Build history of the part. All positions in model axes, mm. A direction names the side the tool comes from. Round coordinates to 2 decimals unless told otherwise and drop trailing zeros. Write each loop counter-clockwise with the first axis right and the second up, starting at its lowest first coordinate (ties: lowest second). Pieces come first, ordered by that corner, then holes.
from build123d import *

# Parameters (mm, degrees)
SKETCH1_W               = 17.5
SKETCH1_H               = 80
BOSS_EXTRUDE1_DEPTH     = 100
BOSS_EXTRUDE1_2_DEPTH   = 100
SKETCH2_W               = 70
SKETCH2_H               = 80
BOSS_EXTRUDE2_DEPTH     = 20
CUT_EXTRUDE1_DEPTH      = 145.568322948
CUT_EXTRUDE1_DEPTH_BACK = 145.568322948
SKETCH5_R               = 11.25
CUT_EXTRUDE2_DEPTH      = 145.568322948
CUT_EXTRUDE2_DEPTH_BACK = 145.568322948
SKETCH6_W               = 42.5
SKETCH6_H               = 42.5
CUT_EXTRUDE3_DEPTH      = 7.5
SKETCH7_R               = 1.75
CUT_EXTRUDE4_DEPTH      = 145.568322948
CUT_EXTRUDE4_DEPTH_BACK = 145.568322948
SKETCH8_W               = 42.5
SKETCH8_H               = 42.5
CUT_EXTRUDE5_DEPTH      = 7.5
CUT_EXTRUDE7_DEPTH      = 35
SKETCH10_W              = 47.5
SKETCH10_H              = 15
BOSS_EXTRUDE3_DEPTH     = 47.5
SKETCH11_R              = 11.25
SKETCH11_R_2            = 1.75
CUT_EXTRUDE8_DEPTH      = 142.089510595
SKETCH12_W              = 42.5
SKETCH12_H              = 42.5
CUT_EXTRUDE9_DEPTH      = 5
SKETCH13_R              = 17.5
BOSS_EXTRUDE4_DEPTH     = 20
FILLET1_R               = 10


with BuildPart() as part:
    # Sketch1 → Boss-Extrude1 (new body)
    with BuildSketch(Plane.XY):
        with Locations((-26.25, 0)):
            Rectangle(SKETCH1_W, SKETCH1_H)
    extrude(amount=BOSS_EXTRUDE1_DEPTH)



with BuildPart() as body_2:
    # Sketch1 → Boss-Extrude1 2 (new body)
    with BuildSketch(Plane.XY):
        with Locations((26.25, 0)):
            Rectangle(SKETCH1_W, SKETCH1_H)
    extrude(amount=BOSS_EXTRUDE1_2_DEPTH)


with BuildPart() as part_1:
    add(part.part)

    add(body_2.part)  # Boss-Extrude2 merges body 2
    # Sketch2 → Boss-Extrude2 (add)
    with BuildSketch(Plane.XY.offset(100)):
        Rectangle(SKETCH2_W, SKETCH2_H)
    extrude(amount=BOSS_EXTRUDE2_DEPTH)

    # Sketch3 → Cut-Extrude1 (cut, two sides)
    with BuildSketch(Plane(origin=(35, 0, 0), x_dir=(0, 0, -1), z_dir=(1, 0, 0))) as cut_extrude1_sk:
        with BuildLine():
            ThreePointArc((-55, 0), (-40, -15), (-25, 0))
            Line((-25, 0), (-55, 0))
        make_face()
        with BuildLine():
            Line((-55, 0), (-25, 0))
            ThreePointArc((-25, 0), (-40, 15), (-55, 0))
        make_face()
        with BuildLine():
            ThreePointArc((-40, 40), (-11.715728753, 28.284271247), (0, 0))
            Line((0, 0), (0, 40))
            Line((0, 40), (-40, 40))
        make_face()
        with BuildLine():
            Line((0, -40), (0, 0))
            ThreePointArc((0, 0), (-11.715728753, -28.284271247), (-40, -40))
            Line((-40, -40), (0, -40))
        make_face()
    extrude(amount=CUT_EXTRUDE1_DEPTH, mode=Mode.SUBTRACT)
    extrude(cut_extrude1_sk.sketch, amount=-CUT_EXTRUDE1_DEPTH_BACK, mode=Mode.SUBTRACT)

    # Sketch5 → Cut-Extrude2 (cut, two sides)
    with BuildSketch(Plane.ZY.offset(35)) as cut_extrude2_sk:
        with Locations(Location((90, 0, 0), (0, 0, 270))):
            Circle(SKETCH5_R)
    extrude(amount=CUT_EXTRUDE2_DEPTH, mode=Mode.SUBTRACT)
    extrude(cut_extrude2_sk.sketch, amount=-CUT_EXTRUDE2_DEPTH_BACK, mode=Mode.SUBTRACT)

    # Sketch6 → Cut-Extrude3 (cut)
    with BuildSketch(Plane(origin=(35, 0, 0), x_dir=(0, 0, -1), z_dir=(1, 0, 0))):
        with Locations((-90, 0)):
            Rectangle(SKETCH6_W, SKETCH6_H)
    extrude(amount=-CUT_EXTRUDE3_DEPTH, mode=Mode.SUBTRACT)

    # Sketch7 → Cut-Extrude4 (cut, two sides)
    with BuildSketch(Plane(origin=(35, 0, 0), x_dir=(0, 0, -1), z_dir=(1, 0, 0))) as cut_extrude4_sk:
        with Locations((-105.5, 15.5)):
            Circle(SKETCH7_R)
        with Locations((-74.5, 15.5)):
            Circle(SKETCH7_R)
        with Locations((-74.5, -15.5)):
            Circle(SKETCH7_R)
        with Locations((-105.5, -15.5)):
            Circle(SKETCH7_R)
    extrude(amount=CUT_EXTRUDE4_DEPTH, mode=Mode.SUBTRACT)
    extrude(cut_extrude4_sk.sketch, amount=-CUT_EXTRUDE4_DEPTH_BACK, mode=Mode.SUBTRACT)

    # Sketch8 → Cut-Extrude5 (cut)
    with BuildSketch(Plane.ZY.offset(35)):
        with Locations((90, 0)):
            Rectangle(SKETCH8_W, SKETCH8_H)
    extrude(amount=-CUT_EXTRUDE5_DEPTH, mode=Mode.SUBTRACT)

    # Sketch9 → Cut-Extrude7 (cut)
    with BuildSketch(Plane.ZY.offset(-17.5)):
        with BuildLine():
            Line((105.5, 19.25), (95.963116285, 19.25))
            Line((95.963116285, 19.25), (95.963116285, 11.75))
            Line((95.963116285, 11.75), (105.5, 11.75))
            ThreePointArc((105.5, 11.75), (109.25, 15.5), (105.5, 19.25))
        make_face()
        with BuildLine():
            Line((105.5, -11.75), (95.963116285, -11.75))
            Line((95.963116285, -11.75), (95.963116285, -19.25))
            Line((95.963116285, -19.25), (105.5, -19.25))
            ThreePointArc((105.5, -19.25), (109.25, -15.5), (105.5, -11.75))
        make_face()
    extrude(amount=CUT_EXTRUDE7_DEPTH, mode=Mode.SUBTRACT)

    # Sketch10 → Boss-Extrude3 (add)
    with BuildSketch(Plane(origin=(0, 40, 0), x_dir=(1, 0, 0), z_dir=(0, 1, 0))):
        with Locations((0, -112.5)):
            Rectangle(SKETCH10_W, SKETCH10_H)
    extrude(amount=BOSS_EXTRUDE3_DEPTH)

    # Sketch11 → Cut-Extrude8 (cut, through all)
    with BuildSketch(Plane(origin=(0, 0, 105), x_dir=(-1, 0, 0), z_dir=(0, 0, -1))):
        with Locations((0, 63.75)):
            Circle(SKETCH11_R)
        with Locations((15.5, 79.25)):
            Circle(SKETCH11_R_2)
        with Locations((15.5, 48.25)):
            Circle(SKETCH11_R_2)
        with Locations((-15.5, 48.25)):
            Circle(SKETCH11_R_2)
        with Locations((-15.5, 79.25)):
            Circle(SKETCH11_R_2)
    extrude(amount=-CUT_EXTRUDE8_DEPTH, mode=Mode.SUBTRACT)

    # Sketch12 → Cut-Extrude9 (cut)
    with BuildSketch(Plane(origin=(0, 0, 105), x_dir=(-1, 0, 0), z_dir=(0, 0, -1))):
        with Locations((0, 63.75)):
            Rectangle(SKETCH12_W, SKETCH12_H)
    extrude(amount=-CUT_EXTRUDE9_DEPTH, mode=Mode.SUBTRACT)

    # Sketch13 → Boss-Extrude4 (add)
    with BuildSketch(Plane.XY.offset(120)):
        with Locations(Location((0, 0, 0), (0, 0, 180))):
            Circle(SKETCH13_R)
    extrude(amount=BOSS_EXTRUDE4_DEPTH)

    # Fillet1
    fillet1_edges = [part_1.edges().sort_by_distance(p)[0] for p in [
        (-17.5, -40, 70),
        (-17.5, 40, 70),
        (17.5, 0, 0),
        (-17.5, 0, 0),
        (17.5, -40, 70),
        (17.5, 40, 70),
    ]]
    fillet(fillet1_edges, radius=FILLET1_R)


solid = part_1.part
1) Which spindle directions (+Z, -Z, +X, -X, +Y, -Y) get a long thin tool onto all of the face, cutting with end or side? Do faces 4 (the cylindrical face through (-20.51, 37.15, 69.58)), 5 (the cylindrical face through (0.25, 15.42, 109.25)), 6 (the flat face through (31, 0, 111.25)), 7 (the flat face through (-2, 87, 105)). Say none if no direction does.
Results:
face 4: -Z, +Y
face 5: -Z
face 6: +X
face 7: -Z, +X, -X, +Y
2) Mould opens along Z. For faces 1 (the flat face through (0, 85, 107)), 2 (the cylindrical face through (0.25, -15.58, 109.25)), 3 (the flat face through (-27.5, -9, 99)) say: released by +Z, released by -Z, zero draft, split by the parting line, or undercut.
Results:
face 1: zero draft
face 2: released by -Z
face 3: undercut
3) Slice it at D-D (x = -15.5). Count the separate pieces of the cut face and the enclosed holes in it, plus the area to 3 significant figures.
Results:
separate pieces: 3
enclosed holes: 0
area: 2,220 mm2
4) Slice it at B-B (x = -30). Write the cut outline in (y, z).
Results:
outline: (-40, 40) arc R40 ccw to (40, 40) - (40, 120) - (-40, 120) - close; hole (-21.25, 68.75) - (21.25, 68.75) - (21.25, 111.25) - (-21.25, 111.25) - close; hole circle Ø30 at (0, 40)
5) Pin check, flat tips, straight feed: pin 1 Ø10 at (x, y) = (13.5, 67.5) entering from +Z; pin 2 Ø3 at (x, y) = (-2.5, 6) entering from -Z; pin 3 Ø3 at (y, z) = (-15.5, 105.5) entering from +X; pin 4 Ø2 at (x, z) = (-17.5, 93.5) entering from +Y. Stop position of each tip, or through.
Results:
pin 1: stops at z = 120
pin 2: stops at z = 100
pin 3: passes through
pin 4: stops at y = 34.36
6) Wall check: L1, parallel to Y at x = -24, z = 105.5; L2, parallel to Y at x = -15.5, z = 115.5; L3, parallel to Z at x = -20, y = 0.5. Give the ranges that are in metal, low to high.
Results:
L1: y = -40 to -17.25, -13.75 to 13.75, 17.25 to 40
L2: y = -40 to 46.5, 50 to 77.5, 81 to 87.5
L3: z = 3.39 to 25.01, 54.99 to 78.76, 101.24 to 120
7) Slice it at A-A (z = 61). Write the cut outline in (x, y).
Results:
outline: (-35, -40) - (-27.5, -40) arc R10 ccw to (-17.5, -30) - (-17.5, 30) arc R10 ccw to (-27.5, 40) - (-35, 40) - close; (17.5, -30) arc R10 ccw to (27.5, -40) - (35, -40) - (35, 40) - (27.5, 40) arc R10 ccw to (17.5, 30) - close
8) Slice it at C-C (y = 62). Write the cut outline in (x, z), plus the area to 3 significant figures.
Results:
outline: (-23.75, 105) - (-21.25, 105) - (-21.25, 110) - (-11.11, 110) - (-11.11, 120) - (-23.75, 120) - close; (11.11, 110) - (21.25, 110) - (21.25, 105) - (23.75, 105) - (23.75, 120) - (11.11, 120) - close
area: 278 mm2
